```python
from build123d import *

# Parameters (mm, degrees)
F0_W           = 63.5
F0_H           = 76.2
F1_DEPTH       = 3.175
F3_D           = 4.9784
F3_CSINK_D     = 9.1186
F3_CSINK_ANGLE = 82
F5_D           = 7.1374


# Not quite as in the source:
# - a feature names something its author has since deleted; it is built from what else it names


with BuildPart() as f1:
    # F0 (on Right) → F1 (new body)
    with BuildSketch(Plane.YZ):
        Rectangle(F0_W, F0_H)
    extrude(amount=F1_DEPTH)

    # F3 (through all)
    with Locations(Plane.YZ.offset(3.175)):
        with Locations((-22.225, 28.575), (-3.175, -28.575)):
            CounterSinkHole(F3_D / 2, F3_CSINK_D / 2, counter_sink_angle=F3_CSINK_ANGLE)

    # F5 (through all)
    with Locations(Plane.YZ.offset(3.175)):
        with Locations((19.05, 25.4), (19.05, -25.4)):
            Hole(F5_D / 2)


solid = f1.part
```
Build history of the part. All positions in model axes, mm. Coordinates: 2 decimals unless noted, no trailing zeros. Order: outer loops, then holes, each group sorted by start corner. A loop starts at its lowest first (then second) coordinate and runs counter-clockwise, first axis right, second up.
Item 1: Saw through at B-B on x = 1.4. List the corners of the cut face in (y, z) (3 decimals), then the cut area to 3 significant figures.
Filled in:
outline: (-31.75, -38.1) - (31.75, -38.1) - (31.75, 38.1) - (-31.75, 38.1) - close; hole circle Ø6.033 at (-22.225, 28.575); hole circle Ø6.033 at (-3.175, -28.575); hole circle Ø7.137 at (19.05, -25.4); hole circle Ø7.137 at (19.05, 25.4)
area: 4,700 mm2
Item 2: Saw through at A-A on y = 19.05. List the corners of the cut face in (x, z) (3 decimals).
Filled in:
outline: (0, -38.1) - (3.175, -38.1) - (3.175, -28.969) - (0, -28.969) - close; (0, -21.831) - (3.175, -21.831) - (3.175, 21.831) - (0, 21.831) - close; (0, 28.969) - (3.175, 28.969) - (3.175, 38.1) - (0, 38.1) - close
Item 3: Drop flat-ended pins along their axis: pin 1 Ø4.5 at (y, z) = (-22.225, 28.575) entering from +X; pin 2 Ø8 at (y, z) = (19.05, -25.4) entering from +X (3 decimals); pin 3 Ø8 at (y, z) = (-3.175, -28.575) entering from +X. Give the stop position or say it passes through.
Filled in:
pin 1: passes through
pin 2: stops at x = 3.175
pin 3: stops at x = 2.53
Item 4: Drill centre lines: L1, parallel to Z at x = 1.45, y = 19.05; L2, parallel to Y at x = 1.4, z = -27.5; L3, parallel to Z at x = 2.15, y = 17.5. Where is each one in solid material? Low to high.
Filled in:
L1: z = -38.1 to -28.97, -21.83 to 21.83, 28.97 to 38.1
L2: y = -31.75 to -5.99, -0.36 to 16.16, 21.94 to 31.75
L3: z = -38.1 to -28.61, -22.19 to 22.19, 28.61 to 38.1
Item 5: Mould opens along Y. For faces 1 (the flat face through (0, 0, 1)), 2 (the conical face through (0.91, -4.57, -26.39)), 3 (the flat face through (2, 31.75, -1)) say: released by +Y, released by -Y, zero draft, split by the parting line, or undercut.
Filled in:
face 1: zero draft
face 2: undercut
face 3: released by +Y
